Work out the finished part from the listing and answer in its coordinate system (mm). A direction names the side the tool comes from. Round coordinates to 2 decimals unless told otherwise and drop trailing zeros. Write each loop counter-clockwise with the first axis right and the second up, starting at its lowest first coordinate (ties: lowest second). Pieces come first, ordered by that corner, then holes.
1. Flat-ended cylindrical pins translate along their axes: pin 1 Ø3 at (y, z) = (-24.5, 4.5) entering from +X; pin 2 Ø0.7 at (x, z) = (33.5, 5) entering from -Y; pin 3 Ø1.5 at (x, z) = (-36.5, 6) entering from +Y. Find the tip coordinate at first contact, or state that the pin passes through.
2. A tool of negligible diameter and unlimited length cuts with its end or side. For faces 4 (the face through (-34, -12, 5)), 5 (the face through (35, 27, 5)), 6 (the face through (32.6, -5, 5)), 7 (the face through (-45, -27, 5)), from which of +Z, -Z, +X, -X, +Y, -Y can it reach the whole face along a straight path? Write none if from no direction.
3. Find section D-D (y = 17.5). Write down the section's boundary in (x, z).
4. Straight lines are drawn through the part: probe 1 along X at (y, z) = (10.5, 9.5); probe 2 along Y at (x, z) = (-40, 2.5); probe 3 along X at (y, z) = (-27.5, 7). For each, find the intervals that lie inside material, in ascending order.
5. Find section C-C (x = -40). Write down the section's boundary in (y, z).
6. Determine the mould class of faces 1 (the face through (-27.4, -5, 5)), 2 (the face through (20, -32.5, 5)), 3 (the face through (40, 12.5, 5)) for opening direction Y: pulls with the +Y half, pulls with the -Y half, needs draft (parallel to the pull), parting line crosses it, or undercut.
7. Find section A-A (x = 0). Write down the section's boundary in (y, z), and give its area (3 significant figures).
8. Find section B-B (y = 10). Write down the section's boundary in (x, z).
```python
from build123d import *

# Parameters (mm, degrees)
SKETCH1_W           = 100
SKETCH1_H           = 65
BOSS_EXTRUDE1_DEPTH = 10
SKETCH2_R           = 1.5
SKETCH2_R_2         = 6.25
CUT_EXTRUDE1_DEPTH  = 61.466933112
SKETCH3_W           = 10
SKETCH3_H           = 12
CUT_EXTRUDE2_DEPTH  = 61.466933112
LPATTERN1_COUNT     = 4
LPATTERN1_PITCH     = 20
SKETCH4_W           = 5
SKETCH4_H           = 12
CUT_EXTRUDE3_DEPTH  = 61.466933112
SKETCH6_R           = 2.5
SKETCH6_W           = 10
SKETCH6_H           = 10
CUT_EXTRUDE4_DEPTH  = 61.466933112


with BuildPart() as part:
    # Sketch1 → Boss-Extrude1 (new body)
    with BuildSketch(Plane.XY):
        Rectangle(SKETCH1_W, SKETCH1_H)
    extrude(amount=BOSS_EXTRUDE1_DEPTH)

    # Sketch2 → Cut-Extrude1 (cut, through all)
    with BuildSketch(Plane.XY.offset(10)):
        with Locations((-15.75, 12.5)):
            Circle(SKETCH2_R)
        with Locations((-7.875, 26.13990011)):
            Circle(SKETCH2_R)
        with Locations((7.875, 26.13990011)):
            Circle(SKETCH2_R)
        with Locations((15.75, 12.5)):
            Circle(SKETCH2_R)
        with Locations((7.875, -1.13990011)):
            Circle(SKETCH2_R)
        with Locations((-7.875, -1.13990011)):
            Circle(SKETCH2_R)
        with Locations((0, 19.5)):
            Circle(SKETCH2_R_2)
    extrude(amount=-CUT_EXTRUDE1_DEPTH, mode=Mode.SUBTRACT)

    # Sketch3 → Cut-Extrude2 (cut, through all)
    with BuildSketch(Plane.XY.offset(10)):
        with Locations((-30, -26.5)):
            Rectangle(SKETCH3_W, SKETCH3_H)
    cut_extrude2 = extrude(amount=-CUT_EXTRUDE2_DEPTH, mode=Mode.SUBTRACT)

    # LPattern1: Cut-Extrude2 ×4
    with Locations(*[(i * LPATTERN1_PITCH, 0, 0) for i in range(1, LPATTERN1_COUNT)]):
        add(cut_extrude2, mode=Mode.SUBTRACT)

    # Sketch4 → Cut-Extrude3 (cut, through all)
    with BuildSketch(Plane.XY.offset(10)):
        with Locations((-47.5, -26.5)):
            Rectangle(SKETCH4_W, SKETCH4_H)
        Polygon((-34, -9.5), (-34, -15.5), (-32.6, -15.5), (-32.6, -20.5), (-27.4, -20.5), (-27.4, -15.5), (-26, -15.5), (-26, -9.5), (-27.4, -9.5), (-27.4, -0.5), (-32.6, -0.5), (-32.6, -9.5), align=None)
    cut_extrude3 = extrude(amount=-CUT_EXTRUDE3_DEPTH, mode=Mode.SUBTRACT)

    # Sketch6 → Cut-Extrude4 (cut, through all)
    with BuildSketch(Plane.XY.offset(10)):
        with Locations((-40, 17.5)):
            Circle(SKETCH6_R)
        with Locations((-40, 27.5)):
            Rectangle(SKETCH6_W, SKETCH6_H)
        with Locations((-40, 7.5)):
            Rectangle(SKETCH6_W, SKETCH6_H)
    cut_extrude4 = extrude(amount=-CUT_EXTRUDE4_DEPTH, mode=Mode.SUBTRACT)

    # Mirror1: Cut-Extrude3, Cut-Extrude4 across plane
    add(cut_extrude3.mirror(Plane(origin=(0, 0, 0), x_dir=(0, 0, 1), z_dir=(1, 0, 0))), mode=Mode.SUBTRACT)
    add(cut_extrude4.mirror(Plane(origin=(0, 0, 0), x_dir=(0, 0, 1), z_dir=(1, 0, 0))), mode=Mode.SUBTRACT)


solid = part.part
```
Worked answers:
1. pin 1: stops at x = 45
1. pin 2: stops at y = -20.5
1. pin 3: stops at y = 22.5
2. face 4: +Z, -Z
2. face 5: +Z, -Z, +Y
2. face 6: +Z, -Z, -Y
2. face 7: +Z, -Z, -X, -Y
3. outline: (-50, 0) - (-42.5, 0) - (-42.5, 10) - (-50, 10) - close; (-37.5, 0) - (-5.92, 0) - (-5.92, 10) - (-37.5, 10) - close; (5.92, 0) - (37.5, 0) - (37.5, 10) - (5.92, 10) - close; (42.5, 0) - (50, 0) - (50, 10) - (42.5, 10) - close
4. probe 1: x = -50 to -45, -35 to 35, 45 to 50
4. probe 2: y = -32.5 to 2.5, 12.5 to 15, 20 to 22.5
4. probe 3: x = -45 to -35, -25 to -15, -5 to 5, 15 to 25, 35 to 45
5. outline: (-32.5, 0) - (2.5, 0) - (2.5, 10) - (-32.5, 10) - close; (12.5, 0) - (15, 0) - (15, 10) - (12.5, 10) - close; (20, 0) - (22.5, 0) - (22.5, 10) - (20, 10) - close
6. face 1: needs draft
6. face 2: pulls with the -Y half
6. face 3: undercut
7. outline: (-32.5, 0) - (13.25, 0) - (13.25, 10) - (-32.5, 10) - close; (25.75, 0) - (32.5, 0) - (32.5, 10) - (25.75, 10) - close
7. area: 525 mm2
8. outline: (-50, 0) - (-45, 0) - (-45, 10) - (-50, 10) - close; (-35, 0) - (35, 0) - (35, 10) - (-35, 10) - close; (45, 0) - (50, 0) - (50, 10) - (45, 10) - close
